```python
from build123d import *

# Parameters (mm, degrees)
F0_R     = 2
F0_R_2   = 16
F0_R_3   = 12
F1_DEPTH = 15
F2_T     = -1.3
F3_R     = 16
F4_DEPTH = 13.7


with BuildPart() as f1:
    # F0 (on Right) → F1 (new body)
    with BuildSketch(Plane.YZ):
        with BuildLine():
            Line((0, 27.04), (-25, 27.04))
            Line((-25, 27.04), (-25, 7.04))
            Line((-25, 7.04), (-23.5, 7.04))
            ThreePointArc((-23.5, 7.04), (-22.6936430136, 6.6314291255), (-22.5461939854, 5.7395768209))
            ThreePointArc((-22.5461939854, 5.7395768209), (-23.4283913263, -4.5038147219), (-19.878453039, -14.152818847))
            ThreePointArc((-19.878453039, -14.152818847), (-19.5668833751, -15.3965751397), (-20.074631189, -16.5739440406))
            Line((-20.074631189, -16.5739440406), (-20.6000079963, -17.1569339704))
            ThreePointArc((-20.6000079963, -17.1569339704), (-20.3430660296, -22.1000079963), (-15.3999920037, -21.8430660296))
            Line((-15.3999920037, -21.8430660296), (-15.2364696163, -21.6616116833))
            ThreePointArc((-15.2364696163, -21.6616116833), (-14.0211573422, -21.0188707984), (-12.6780712141, -21.3125022359))
            ThreePointArc((-12.6780712141, -21.3125022359), (-6.6017257113, -24.0594120315), (0, -25))
            ThreePointArc((0, -25), (18.0346887969, -17.7360763487), (26, 0))
            ThreePointArc((26, 0), (24.8756586881, 8.6516449625), (20.9547141799, 16.4453153497))
            ThreePointArc((20.9547141799, 16.4453153497), (20.5678212068, 17.7298278052), (21.0796574448, 18.969860904))
            Line((21.0796574448, 18.969860904), (22.6000079963, 20.6569339704))
            ThreePointArc((22.6000079963, 20.6569339704), (22.3430660296, 25.6000079963), (17.3999920037, 25.3430660296))
            Line((17.3999920037, 25.3430660296), (15.9178980328, 23.6984447825))
            ThreePointArc((15.9178980328, 23.6984447825), (14.7273428061, 23.0592399542), (13.4020450466, 23.3230398953))
            ThreePointArc((13.4020450466, 23.3230398953), (6.9539665632, 26.0935467981), (0, 27.04))
        make_face()
        with Locations((-18, -19.5)):
            Circle(F0_R, mode=Mode.SUBTRACT)
        Circle(F0_R_2, mode=Mode.SUBTRACT)
        with Locations((20, 23)):
            Circle(F0_R, mode=Mode.SUBTRACT)
        Circle(F0_R_2)
        Circle(F0_R_3, mode=Mode.SUBTRACT)
        Circle(F0_R_3)
    extrude(amount=F1_DEPTH)

    # F2
    f2_openings = [f1.faces().sort_by_distance(p)[0] for p in [
        (7.5, -25, 17.04),
    ]]
    offset(amount=F2_T, openings=f2_openings)

    # F3 (on face) → F4 (cut, through all)
    with BuildSketch(Plane.YZ.offset(15)):
        Circle(F3_R)
    extrude(amount=-F4_DEPTH, mode=Mode.SUBTRACT)


solid = f1.part
```
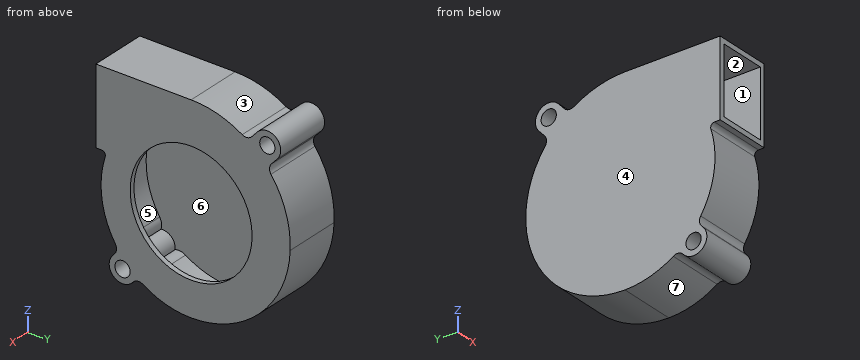
Design review of the part built by this model. Coordinates are the model's own, in mm. Face numbers are marked on the shaded views. A direction names the side the tool comes from. Coordinates: 2 decimals unless noted, no trailing zeros. Order: outer loops, then holes, each group sorted by start corner. A loop starts at its lowest first (then second) coordinate and runs counter-clockwise, first axis right, second up.
1) Take a section at B-B, the plane y = 7. Give the boundary of the cut face in (x, z).
2) Mouldability with a two-part tool opening along Z and no side actions: class the marked faces 4, 5, 6 and 7 as +Z half, -Z half, draft (parallel to the pull), parting line (faces both ways), or undercut.
3) Wall thickness on line 1 along Z through (x, y) = (12, -18); line 2 along X through (y, z) = (-14.5, 8.5); line 3 along Y through (x, z) = (1.75, -18.5): over which ranges is each line inside the solid? List them lowest first.
4) Take a section at D-D, the plane y = 14. Give the boundary of the cut face in (x, z), and give its area (3 significant figures).
5) Take a section at C-C, the plane x = 6.5. State how many separate pieces and enclosed holes the cut face has, and give its area (3 significant figures).
6) Take a section at A-A, the plane z = 9. Give the boundary of the cut face in (x, y), and give its area (3 significant figures).
7) For the marked faces 1, 2 and 3, list the 3-axis set-ups (+Z, -Z, +X, -X, +Y, -Y) from which the entire face can be reached by the end or side of a thin tool; tool diameter is ignored.
8) Clearance check with flat-ended pins moving along their axes: pin 1 (3 mm diameter, centred on y = 3, z = -8, fed in from +X); pin 2 (1.5 mm diameter, centred on x = 10.5, z = -0.5, fed in from +Y); pin 3 (6 mm diameter, centred on x = 13.5, y = -11, fed in from -Z). State where each tip first meets the part, or that it passes through.
Returned:
1. outline: (0, -24.04) - (15, -24.04) - (15, -14.39) - (13.7, -14.39) - (13.7, -22.69) - (1.3, -22.69) - (1.3, 24.73) - (13.7, 24.73) - (13.7, 14.39) - (15, 14.39) - (15, 26.08) - (0, 26.08) - close
2. face 4: draft
2. face 5: undercut
2. face 6: undercut
2. face 7: -Z half
3. line 1: z = -23 to -21.5, -17.5 to -16.2, 25.74 to 27.04
3. line 2: x = 0 to 1.3, 13.7 to 15
3. line 3: y = -21.35 to -19.73, -16.27 to -14.86, 15.17 to 17.2
4. outline: (0, -20.91) - (15, -20.91) - (15, -7.75) - (13.7, -7.75) - (13.7, -19.35) - (1.3, -19.35) - (1.3, 21.77) - (13.7, 21.77) - (13.7, 7.75) - (15, 7.75) - (15, 23.08) - (0, 23.08) - close
4. area: 130 mm2
5. separate pieces: 1
5. enclosed holes: 2
5. area: 239 mm2
6. outline: (0, -25) - (1.3, -25) - (1.3, 23.4) - (13.7, 23.4) - (13.7, 13.23) - (15, 13.23) - (15, 24.77) - (0, 24.77) - close; (13.7, -25) - (15, -25) - (15, -13.23) - (13.7, -13.23) - close
6. area: 112 mm2
7. face 1: none
7. face 2: -Y
7. face 3: +Z, +X, -X
8. pin 1: stops at x = 1.3
8. pin 2: stops at y = 26.01
8. pin 3: stops at z = -23.61
